Check sheet for the modelled part. Datum: model origin and axes. Units: mm. Face numbers are marked on the shaded views. A direction names the side the tool comes from. Coordinates: 2 decimals unless noted, no trailing zeros. Write each loop counter-clockwise with the first axis right and the second up, starting at its lowest first coordinate (ties: lowest second). Pieces come first, ordered by that corner, then holes. Notation, with made-up numbers: M 52,0.25 L 79,0.25 A25 ccw 79,35.25 Z; hole C -8.75,-23 d9. An arc over 180 degrees is marked long. Answer as CSV lines item,"result". Start each with the question number.
Q1. Sectioned sample at B-B, the plane y = -6.25. Record the cut outline in (x, z).
Q2. Sectioned sample at D-D, the plane x = 28.5. Record the cut outline in (y, z).
Q3. Access from +Z, -Z, +X, -X, +Y, -Y to the whole of each face (thin tool, end or side, straight path). Record for the marked faces 4 and 5.
Q4. Sectioned sample at C-C, the plane y = 11. Record the cut outline in (x, z), then the cut area to 3 significant figures.
Q5. Mould release check, pull along Z, two halves, no side actions. Record for the marked faces 1, 2 and 3: pulls with the +Z half, pulls with the -Z half, needs draft (parallel to the pull), parting line crosses it, or undercut.
Q6. Sectioned sample at A-A, the plane z = 0. Record the cut outline in (x, y), then the cut area to 3 significant figures.
Q7. Depth check by flat-ended pin: pin 1 Ø4 at (x, y) = (-31, -6) entering from +Z; pin 2 Ø8 at (x, y) = (-27, 1.5) entering from +Z; pin 3 Ø20.5 at (x, z) = (0, 0) entering from -Y. Enter the tip coordinate at first touch or a pass-through.
Q8. Thickness scan on line 1 along Z through (x, y) = (2, 7); line 2 along Z through (x, y) = (0, 6.25); line 3 along X through (y, z) = (-8.75, 8). Record the ranges inside material, lowest first. Write a range as from..to.
from build123d import *

# Parameters (mm, degrees)
SKETCH2_R                = 10
BOSS_EXTRUDE1_DEPTH      = 45
BOSS_EXTRUDE1_DEPTH_BACK = 45
SKETCH1_R                = 25.4
SKETCH1_R_2              = 12.7
BOSS_EXTRUDE2_DEPTH      = 12.7
BOSS_EXTRUDE2_DEPTH_BACK = 12.7


with BuildPart() as part:
    # Sketch2 → Boss-Extrude1 (new body, two sides)
    with BuildSketch(Plane(origin=(0, 0, 0), x_dir=(0, 0, -1), z_dir=(1, 0, 0))) as boss_extrude1_sk:
        Circle(SKETCH2_R)
    extrude(amount=BOSS_EXTRUDE1_DEPTH)
    extrude(boss_extrude1_sk.sketch, amount=-BOSS_EXTRUDE1_DEPTH_BACK)

    # Sketch1 → Boss-Extrude2 (add, two sides)
    with BuildSketch(Plane(origin=(0, 0, 0), x_dir=(1, 0, 0), z_dir=(0, 1, 0))) as boss_extrude2_sk:
        Circle(SKETCH1_R)
        Circle(SKETCH1_R_2, mode=Mode.SUBTRACT)
    extrude(amount=BOSS_EXTRUDE2_DEPTH)
    extrude(boss_extrude2_sk.sketch, amount=-BOSS_EXTRUDE2_DEPTH_BACK)


solid = part.part
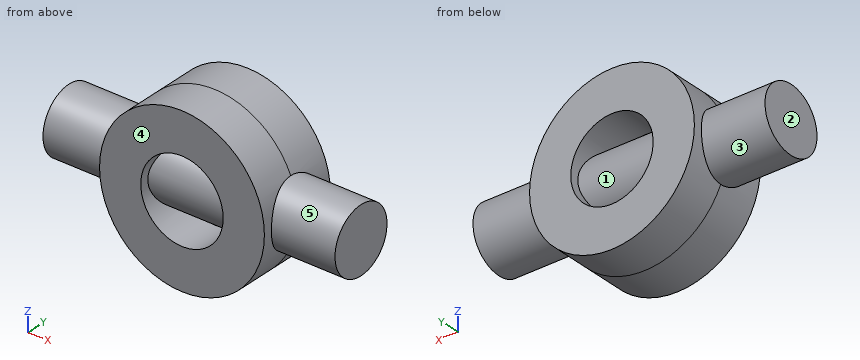
Output:
1,outline,"M -45,-7.81 L -24.17,-7.81 A25.4 ccw 24.17,-7.81 L 45,-7.81 L 45,7.81 L 24.17,7.81 A25.4 ccw -24.17,7.81 L -45,7.81 Z; hole M -10.02,-7.81 A12.7 ccw 10.02,-7.81 Z; hole M -10.02,7.81 L 10.02,7.81 A12.7 ccw Z"
2,outline,"C 0,0 d20"
3,face 4,"+Z, -Z, +X, -X, -Y"
3,face 5,"+X"
4,outline,"C 0,0 d50.8; hole C 0,0 d25.4"
4,area,"1,520 mm^2"
5,face 1,"undercut"
5,face 2,"needs draft"
5,face 3,"parting line crosses it"
6,outline,"M -45,-10 L -25.4,-10 L -25.4,-12.7 L -12.7,-12.7 L -12.7,-10 L 12.7,-10 L 12.7,-12.7 L 25.4,-12.7 L 25.4,-10 L 45,-10 L 45,10 L 25.4,10 L 25.4,12.7 L 12.7,12.7 L 12.7,10 L -12.7,10 L -12.7,12.7 L -25.4,12.7 L -25.4,10 L -45,10 Z"
6,area,"1,940 mm^2"
7,pin 1,"stops at z = 9.17"
7,pin 2,"stops at z = 10.78"
7,pin 3,"stops at y = -10"
8,line 1,"z = -25.32..-12.54, -7.14..7.14, 12.54..25.32"
8,line 2,"z = -25.4..-12.7, -7.81..7.81, 12.7..25.4"
8,line 3,"x = -24.11..-9.86, 9.86..24.11"
